Could you check a few things on this model? Use its own coordinates, in mm. A direction names the side the tool comes from. Coordinates: 2 decimals unless noted, no trailing zeros. Order: outer loops, then holes, each group sorted by start corner. A loop starts at its lowest first (then second) coordinate and runs counter-clockwise, first axis right, second up. Notation, with made-up numbers: (-12, 53.25) -> (14, 53.25) arc R18 cw to (14, 58.25) -> close; hole circle Ø1 at (14, -12). An arc over 180 degrees is marked (long way). Put each result on its own line as item: value. Start each with the question number.
Q1. If we section it at D-D (y = 11): Please give me the cut outline in (x, z) (3 decimals).
Q2. Will these pins go through, and if not, where does the flat tip stop? pin 1 (5 mm diameter, centred on x = -92.35, y = 160.4, fed in from -Z) (3 decimals); pin 2 (4.5 mm diameter, centred on x = 0, y = 146.05, fed in from +Z); pin 3 (8 mm diameter, centred on x = 28.5, z = 1, fed in from +Y) (3 decimals).
Q3. If we section it at A-A (y = 108): Please give me the cut outline in (x, z) (3 decimals).
Q4. If we section it at C-C (z = -40): Please give me the cut outline in (x, y) (3 decimals).
Q5. Please list where these lines run through material, in increasing order: line 1 along X through (y, z) = (146.05, 23.4); line 2 along Y through (x, z) = (76.2, 22.7) (3 decimals); line 3 along Y through (x, z) = (35.5, -31) (3 decimals).
Q6. If we section it at B-B (x = 19): Please give me the cut outline in (y, z) (3 decimals).
Q7. For faces 1 (the face through (89.09, -23.79, -69.84)), 2 (the face through (1, 56, 22.225)), which set-ups out of +Z, -Z, +X, -X, +Y, -Y let a thin tool reach every point of the face, with its end or its side?
from build123d import *

# Parameters (mm, degrees)
BASE_FLANGE1_DEPTH                                = 102.87
SKETCH6_W                                         = 6.35
SKETCH6_H                                         = 99.06
CUT_EXTRUDE1_DEPTH                                = 10.16
FILLET1_R                                         = 21.336
FILLET2_R                                         = 12.7
SKETCH8_W                                         = 177.8
SKETCH8_H                                         = 66.675
CUT_EXTRUDE2_DEPTH                                = 10.16
CSK_FOR_6_FLAT_HEAD_MACHINE_SCREW_100_D           = 3.7973
CSK_FOR_6_FLAT_HEAD_MACHINE_SCREW_100_CSINK_D     = 7.0866
CSK_FOR_6_FLAT_HEAD_MACHINE_SCREW_100_CSINK_ANGLE = 100
CSK_FOR_6_FLAT_HEAD_MACHINE_SCREW_2_D             = 3.7973
CSK_FOR_6_FLAT_HEAD_MACHINE_SCREW_2_CSINK_D       = 7.0866
CSK_FOR_6_FLAT_HEAD_MACHINE_SCREW_2_CSINK_ANGLE   = 100


# Sheet-metal steps are written as plain solids
with BuildPart() as part:
    # Sketch1 → Base-Flange1 (new, symmetric)
    with BuildSketch(Plane.YZ):
        with BuildLine():
            Line((-25.4, -73.66), (-25.4, 19.05))
            ThreePointArc((-25.4, 19.05), (-23.540128061, 23.540128061), (-19.05, 25.4))
            Line((-19.05, 25.4), (171.45, 25.4))
            Line((171.45, 25.4), (171.45, 22.225))
            Line((171.45, 22.225), (-19.05, 22.225))
            ThreePointArc((-19.05, 22.225), (-21.29506403, 21.29506403), (-22.225, 19.05))
            Line((-22.225, 19.05), (-22.225, -73.66))
            Line((-22.225, -73.66), (-25.4, -73.66))
        make_face()
    extrude(amount=BASE_FLANGE1_DEPTH, both=True)

    # Sketch6 → Cut-Extrude1 (cut)
    with BuildSketch(Plane.YZ.offset(102.87)):
        with Locations((-22.225, -24.13)):
            Rectangle(SKETCH6_W, SKETCH6_H)
    cut_extrude1 = extrude(amount=-CUT_EXTRUDE1_DEPTH, mode=Mode.SUBTRACT)

    # Mirror1: Cut-Extrude1 across plane
    add(cut_extrude1.mirror(Plane(origin=(0, 0, 0), x_dir=(0, 0, 1), z_dir=(1, 0, 0))), mode=Mode.SUBTRACT)

    # Fillet1
    fillet1_edges = [part.edges().sort_by_distance(p)[0] for p in [
        (102.87, 171.45, 23.8125),
        (-102.87, 171.45, 23.8125),
    ]]
    fillet(fillet1_edges, radius=FILLET1_R)

    # Fillet2
    fillet2_edges = [part.edges().sort_by_distance(p)[0] for p in [
        (92.71, -23.8125, -73.66),
        (-92.71, -23.8125, -73.66),
    ]]
    fillet(fillet2_edges, radius=FILLET2_R)

    # Sketch8 → Cut-Extrude2 (cut)
    with BuildSketch(Plane.XY.offset(25.4)):
        with Locations((0, 100.0125)):
            Rectangle(SKETCH8_W, SKETCH8_H)
    extrude(amount=-CUT_EXTRUDE2_DEPTH, mode=Mode.SUBTRACT)

    # CSK for _6 Flat Head Machine Screw _100 (through all)
    with Locations(Plane.XY.offset(25.4)):
        with Locations((-76.2, 146.05), (0, 146.05), (76.2, 146.05), (76.2, 53.975), (0, 53.975), (-76.2, 53.975)):
            CounterSinkHole(CSK_FOR_6_FLAT_HEAD_MACHINE_SCREW_100_D / 2, CSK_FOR_6_FLAT_HEAD_MACHINE_SCREW_100_CSINK_D / 2, counter_sink_angle=CSK_FOR_6_FLAT_HEAD_MACHINE_SCREW_100_CSINK_ANGLE)

    # CSK for _6 Flat Head Machine Screw _ 2 (through all)
    with Locations(Plane.XY.offset(25.4)):
        with Locations((92.4814, 160.8074), (95.4278, 92.583), (95.4278, -6.223), (-95.758, 1.016), (-95.758, 85.344), (-92.3544, 160.401), (3.2512, 163.6268)):
            CounterSinkHole(CSK_FOR_6_FLAT_HEAD_MACHINE_SCREW_2_D / 2, CSK_FOR_6_FLAT_HEAD_MACHINE_SCREW_2_CSINK_D / 2, counter_sink_angle=CSK_FOR_6_FLAT_HEAD_MACHINE_SCREW_2_CSINK_ANGLE)


solid = part.part
The answers:
1. outline: (-102.87, 22.225) -> (102.87, 22.225) -> (102.87, 25.4) -> (-102.87, 25.4) -> close
2. pin 1: z = 22.225
2. pin 2: z = 24.31
2. pin 3: y = -22.225
3. outline: (-102.87, 22.225) -> (-88.9, 22.225) -> (-88.9, 25.4) -> (-102.87, 25.4) -> close; (88.9, 22.225) -> (102.87, 22.225) -> (102.87, 25.4) -> (88.9, 25.4) -> close
4. outline: (-92.71, -25.4) -> (92.71, -25.4) -> (92.71, -22.225) -> (-92.71, -22.225) -> close
5. line 1: -102.87 to -78.1, -74.3 to -1.9, 1.9 to 74.3, 78.1 to 102.87
5. line 2: -24.246 to 52.076, 55.874 to 66.675, 133.35 to 144.151, 147.949 to 171.45
5. line 3: -25.4 to -22.225
6. outline: (-25.4, -73.66) -> (-22.225, -73.66) -> (-22.225, 19.05) arc R3.175 cw to (-19.05, 22.225) -> (66.675, 22.225) -> (66.675, 25.4) -> (-19.05, 25.4) arc R6.35 ccw to (-25.4, 19.05) -> close; (133.35, 22.225) -> (171.45, 22.225) -> (171.45, 25.4) -> (133.35, 25.4) -> close
7. face 1: -Z, +X, +Y, -Y
7. face 2: -Z, +X, -X, +Y
